Part print with two shaded views. Sizes in mm from the minimum x, y, z corner. A direction names the side the tool comes from. Give positions to 0.01 mm unless a question says otherwise; leave off trailing zeros. Order: outer loops, then holes, each group sorted by start corner. A loop starts at its lowest first (then second) coordinate and runs counter-clockwise, first axis right, second up. Notation, with made-up numbers: (-9, 81) -> (26, 81) arc R23 cw to (26, 114) -> close; hole circle Ø7 at (81, -26). An arc over 180 degrees is marked (long way). Write item = value, one per line. Start each with the question number.
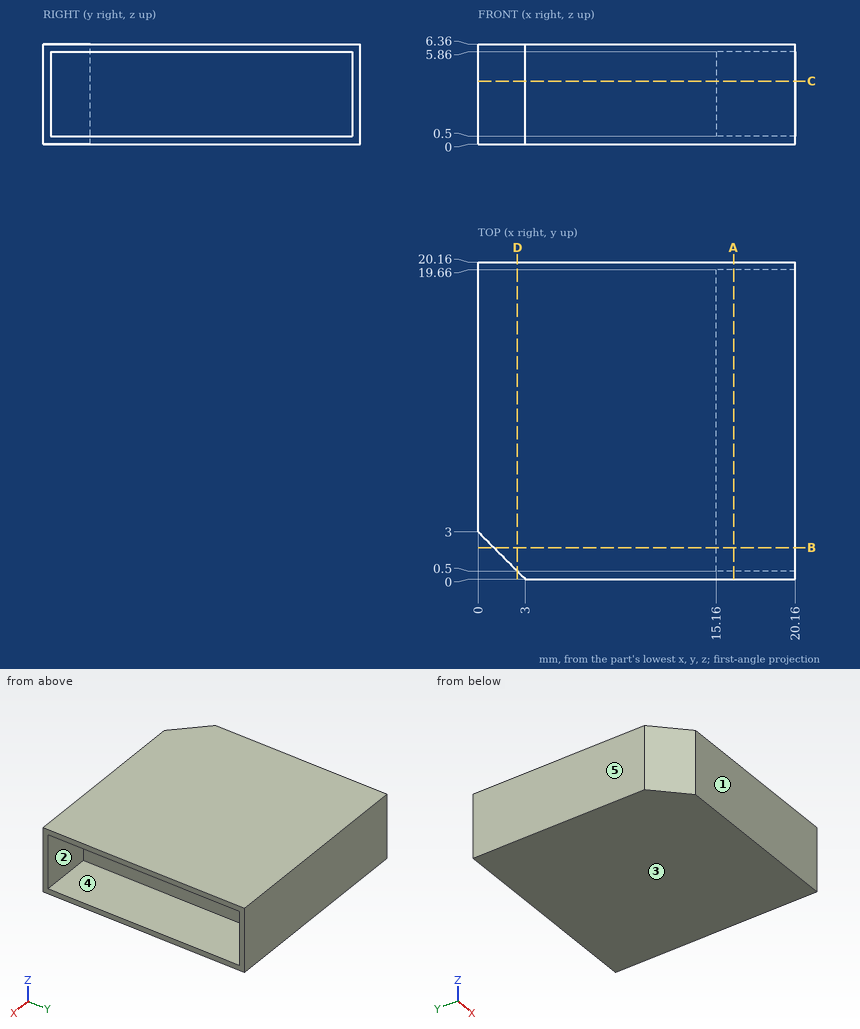
(1) Cut at B-B, the plane y = 2. Give the cut face in (x, z), plus the area to 3 significant figures.
(2) Wall check: line 1 (Y direction, x = 18, z = 2); line 2 (Z direction, x = 19.75, y = 2.5); line 3 (Y direction, x = 2.5, z = 1.5). Give the ranges that are in metal, low to high. Write a range as [from, to].
(3) Flat gauge pin, fed straight in: P1, Ø1.6, axis at y = 14, z = 3.5, coming from the +X side. Where does the tip first touch, or does it go through?
(4) Cut at C-C, the plane z = 4. Give the cut face in (x, y), plus the area to 3 significant figures.
(5) Cut at D-D, the plane x = 2.5. Give the cut face in (y, z), plus the area to 3 significant figures.
(6) Mould opens along Z. For the marked faces 3, 4 and 5 say: released by +Z, released by -Z, zero draft, split by the parting line, or undercut.
(7) 3-axis set-ups, long thin cutter, end or side, ignore diameter. For the marked faces 1 and 2: which of +Z, -Z, +X, -X, +Y, -Y reach the whole face in a straight line?
(8) Cut at A-A, the plane x = 16.25. Give the cut face in (y, z), plus the area to 3 significant figures.
Results:
q1.outline = (1, 0) -> (20.16, 0) -> (20.16, 0.5) -> (15.16, 0.5) -> (15.16, 5.86) -> (20.16, 5.86) -> (20.16, 6.36) -> (1, 6.36) -> close
q1.area = 95.1 mm2
q2.line_1 = [0, 0.5], [19.66, 20.16]
q2.line_2 = [0, 0.5], [5.86, 6.36]
q2.line_3 = [0.5, 20.16]
q3.P1 = 15.16
q4.outline = (0, 3) -> (3, 0) -> (20.16, 0) -> (20.16, 0.5) -> (15.16, 0.5) -> (15.16, 19.66) -> (20.16, 19.66) -> (20.16, 20.16) -> (0, 20.16) -> close
q4.area = 306 mm2
q5.outline = (0.5, 0) -> (20.16, 0) -> (20.16, 6.36) -> (0.5, 6.36) -> close
q5.area = 125 mm2
q6.face_3 = released by -Z
q6.face_4 = undercut
q6.face_5 = zero draft
q7.face_1 = +Z, -Z, +X, -X, -Y
q7.face_2 = +X
q8.outline = (0, 0) -> (20.16, 0) -> (20.16, 6.36) -> (0, 6.36) -> close; hole (0.5, 0.5) -> (19.66, 0.5) -> (19.66, 5.86) -> (0.5, 5.86) -> close
q8.area = 25.5 mm2
